The listing builds one solid part. Answer for the finished solid, in the listing's coordinates (mm). Face numbers are marked on the shaded views. A direction names the side the tool comes from. Coordinates: 2 decimals unless noted, no trailing zeros. Order: outer loops, then holes, each group sorted by start corner. A loop starts at its lowest first (then second) coordinate and runs counter-clockwise, first axis right, second up. Notation, with made-up numbers: M 63,38.25 L 93,38.25 A28 ccw 93,59.25 Z; hole C 80.5,37.25 d4. An arc over 180 degrees is marked long. One line per item, written item: value. Start each with the question number.
Q1. The part is cut by section D-D on x = 14.5. Give the vertices of the cut face in (y, z).
Q2. Determine the mould class of the marked faces 4 and 5 for opening direction X: pulls with the +X half, pulls with the -X half, needs draft (parallel to the pull), parting line crosses it, or undercut.
Q3. The part is cut by section A-A on y = 16. Give the vertices of the cut face in (x, z).
Q4. The part is cut by section C-C on y = -7. Give the vertices of the cut face in (x, z).
Q5. For the marked faces 1, 2 and 3, determine the directions among +Z, -Z, +X, -X, +Y, -Y from which every point of the face is accessible in a straight line to the end or side of a thin tool.
Q6. Straight lines are drawn through the part: line 1 along X through (y, z) = (-11.5, 4.5); line 2 along X through (y, z) = (-27.4, 16); line 3 along Y through (x, z) = (19.5, 6). For each, find the intervals that lie inside material, in ascending order. Write a range as [from, to].
Q7. Each of these flat-tipped pins is pushed along its axis until it touches: pin 1 Ø15.5 at (x, z) = (-20.5, 20) entering from +Y; pin 2 Ø10 at (y, z) = (-9.5, 12) entering from +X; pin 3 Ø2.5 at (x, z) = (16, 14.5) entering from -Y; pin 4 Ø8 at (x, z) = (0, 16) entering from -Y. Where does it stop, or does it pass through?
Q8. The part is cut by section B-B on z = 16. Give the number of separate pieces and of enclosed holes in the cut face, then the cut area to 3 significant figures.
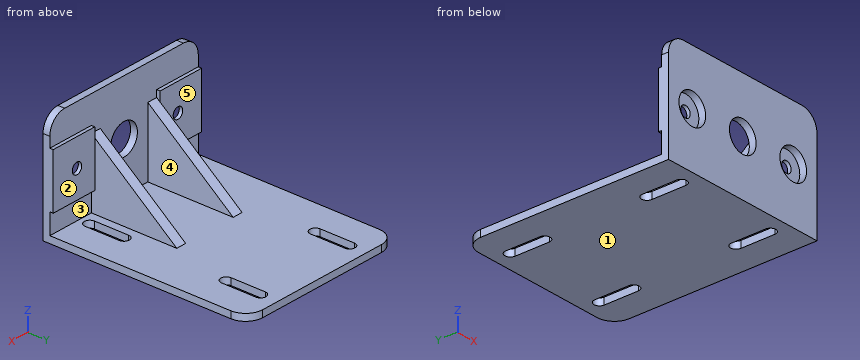
```python
from build123d import *

# Parameters (mm, degrees)
DODANIE_WYCI_GNI_CIE1_DEPTH = 2
WYTNIJ_WYCI_GNI_CIE1_REACH  = 41.102
SZKIC4_W                    = 50
SZKIC4_H                    = 2
DODANIE_WYCI_GNI_CIE2_DEPTH = 30
DODANIE_WYCI_GNI_CIE3_START = -14
DODANIE_WYCI_GNI_CIE3_DEPTH = 3
ZAOKR_GLENIE1_R             = 5
SZKIC7_R                    = 4.5
WYTNIJ_WYCI_GNI_CIE2_DEPTH  = 2
SZKIC8_W                    = 14
SZKIC8_H                    = 16
SZKIC8_R                    = 1.6
DODANIE_WYCI_GNI_CIE4_DEPTH = 1


with BuildPart() as part:
    # Szkic1 → Dodanie-wyci_gni_cie1 (new body)
    with BuildSketch(Plane.XY):
        with BuildLine():
            Line((-25, -30), (25, -30))
            Line((25, -30), (25, 25))
            ThreePointArc((25, 25), (23.535533906, 28.535533906), (20, 30))
            Line((20, 30), (-20, 30))
            ThreePointArc((-20, 30), (-23.535533906, 28.535533906), (-25, 25))
            Line((-25, 25), (-25, -30))
        make_face()
    extrude(amount=DODANIE_WYCI_GNI_CIE1_DEPTH)

    # Szkic2 → Wytnij-wyci_gni_cie1 (cut, up to next)
    with BuildSketch(Plane.XY.offset(2), mode=Mode.PRIVATE) as wytnij_wyci_gni_cie1_sk1:
        with BuildLine():
            Line((-13.4, 25), (-13.4, 15))
            ThreePointArc((-13.4, 15), (-15, 13.4), (-16.6, 15))
            Line((-16.6, 15), (-16.6, 25))
            ThreePointArc((-16.6, 25), (-15, 26.6), (-13.4, 25))
        make_face()
    wytnij_wyci_gni_cie1_tool1 = extrude(wytnij_wyci_gni_cie1_sk1.sketch, amount=-WYTNIJ_WYCI_GNI_CIE1_REACH, mode=Mode.PRIVATE) & part.part
    # Szkic2 → Wytnij-wyci_gni_cie1 (cut, up to next)
    with BuildSketch(Plane.XY.offset(2), mode=Mode.PRIVATE) as wytnij_wyci_gni_cie1_sk2:
        with BuildLine():
            Line((13.4, 25), (13.4, 15))
            ThreePointArc((13.4, 15), (15, 13.4), (16.6, 15))
            Line((16.6, 15), (16.6, 25))
            ThreePointArc((16.6, 25), (15, 26.6), (13.4, 25))
        make_face()
    wytnij_wyci_gni_cie1_tool2 = extrude(wytnij_wyci_gni_cie1_sk2.sketch, amount=-WYTNIJ_WYCI_GNI_CIE1_REACH, mode=Mode.PRIVATE) & part.part
    # Szkic2 → Wytnij-wyci_gni_cie1 (cut, up to next)
    with BuildSketch(Plane.XY.offset(2), mode=Mode.PRIVATE) as wytnij_wyci_gni_cie1_sk3:
        with BuildLine():
            Line((13.4, -25), (13.4, -15))
            ThreePointArc((13.4, -15), (15, -13.4), (16.6, -15))
            Line((16.6, -15), (16.6, -25))
            ThreePointArc((16.6, -25), (15, -26.6), (13.4, -25))
        make_face()
    wytnij_wyci_gni_cie1_tool3 = extrude(wytnij_wyci_gni_cie1_sk3.sketch, amount=-WYTNIJ_WYCI_GNI_CIE1_REACH, mode=Mode.PRIVATE) & part.part
    # Szkic2 → Wytnij-wyci_gni_cie1 (cut, up to next)
    with BuildSketch(Plane.XY.offset(2), mode=Mode.PRIVATE) as wytnij_wyci_gni_cie1_sk4:
        with BuildLine():
            Line((-13.4, -25), (-13.4, -15))
            ThreePointArc((-13.4, -15), (-15, -13.4), (-16.6, -15))
            Line((-16.6, -15), (-16.6, -25))
            ThreePointArc((-16.6, -25), (-15, -26.6), (-13.4, -25))
        make_face()
    wytnij_wyci_gni_cie1_tool4 = extrude(wytnij_wyci_gni_cie1_sk4.sketch, amount=-WYTNIJ_WYCI_GNI_CIE1_REACH, mode=Mode.PRIVATE) & part.part
    add(wytnij_wyci_gni_cie1_tool1.solids().sort_by_distance((-15, 20, 2))[0], mode=Mode.SUBTRACT)
    add(wytnij_wyci_gni_cie1_tool2.solids().sort_by_distance((15, 20, 2))[0], mode=Mode.SUBTRACT)
    add(wytnij_wyci_gni_cie1_tool3.solids().sort_by_distance((15, -20, 2))[0], mode=Mode.SUBTRACT)
    add(wytnij_wyci_gni_cie1_tool4.solids().sort_by_distance((-15, -20, 2))[0], mode=Mode.SUBTRACT)

    # Szkic4 → Dodanie-wyci_gni_cie2 (add)
    with BuildSketch(Plane.XY.offset(2)):
        with Locations((0, -29)):
            Rectangle(SZKIC4_W, SZKIC4_H)
    extrude(amount=DODANIE_WYCI_GNI_CIE2_DEPTH)


with BuildPart() as body_2:
    # Szkic6 → Dodanie-wyci_gni_cie3 (new body)
    with BuildSketch(Plane.ZY.offset(25).offset(DODANIE_WYCI_GNI_CIE3_START)):
        Polygon((2, -28), (2, -3), (22, -28), align=None)
    dodanie_wyci_gni_cie3 = extrude(amount=-DODANIE_WYCI_GNI_CIE3_DEPTH)


with BuildPart() as part_1:
    add(part.part)

    # Lustro3: Dodanie-wyci_gni_cie3 across plane
    add(dodanie_wyci_gni_cie3.mirror(Plane(origin=(0, 0, 0), x_dir=(0, 0, 1), z_dir=(1, 0, 0))))

    # Zaokr_glenie1
    zaokr_glenie1_edges = [part_1.edges().sort_by_distance(p)[0] for p in [
        (-25, -29, 32),
        (25, -29, 32),
    ]]
    fillet(zaokr_glenie1_edges, radius=ZAOKR_GLENIE1_R)

    # Szkic7 → Wytnij-wyci_gni_cie2 (cut)
    with BuildSketch(Plane.XZ.offset(30)):
        with Locations(Location((0, 16, 0), (0, 0, 270))):
            Circle(SZKIC7_R)
        with Locations(Location((-17, 16, 0), (0, 0, 270))):
            Circle(SZKIC7_R)
        with Locations(Location((17, 16, 0), (0, 0, 270))):
            Circle(SZKIC7_R)
    extrude(amount=-WYTNIJ_WYCI_GNI_CIE2_DEPTH, mode=Mode.SUBTRACT)

    add(body_2.part)  # Dodanie-wyci_gni_cie4 merges body 2
    # Szkic8 → Dodanie-wyci_gni_cie4 (add)
    # profile 1 of 2: a face of its own
    with BuildSketch(Plane(origin=(0, -28, 0), x_dir=(1, 0, 0), z_dir=(0, 1, 0))):
        with Locations((-18, -16)):
            Rectangle(SZKIC8_W, SZKIC8_H)
        with Locations(Location((-17, -16, 0), (0, 0, 270))):
            Circle(SZKIC8_R, mode=Mode.SUBTRACT)
    # profile 2 of 2: a face of its own
    with BuildSketch(Plane(origin=(0, -28, 0), x_dir=(1, 0, 0), z_dir=(0, 1, 0))):
        with Locations((18, -16)):
            Rectangle(SZKIC8_W, SZKIC8_H)
        with Locations(Location((17, -16, 0), (0, 0, 90))):
            Circle(SZKIC8_R, mode=Mode.SUBTRACT)
    extrude(amount=DODANIE_WYCI_GNI_CIE4_DEPTH)


solid = part_1.part
```
Output:
1. outline: M -30,0 L -26.52,0 L -26.52,2 L -28,2 L -28,8 L -27,8 L -27,24 L -28,24 L -28,32 L -30,32 L -30,19.74 L -28,19.74 L -28,12.26 L -30,12.26 Z; M -13.48,0 L 13.48,0 L 13.48,2 L -13.48,2 Z; M 26.52,0 L 30,0 L 30,2 L 26.52,2 Z
2. face 4: undercut
2. face 5: needs draft
3. outline: M -25,0 L -16.6,0 L -16.6,2 L -25,2 Z; M -13.4,0 L 13.4,0 L 13.4,2 L -13.4,2 Z; M 16.6,0 L 25,0 L 25,2 L 16.6,2 Z
4. outline: M -25,0 L 25,0 L 25,2 L 11,2 L 11,5.2 L 8,5.2 L 8,2 L -8,2 L -8,5.2 L -11,5.2 L -11,2 L -25,2 Z
5. face 1: -Z, +X, -X, +Y, -Y
5. face 2: +Z, +X, +Y
5. face 3: +X, +Y
6. line 1: x = [-11, -8], [8, 11]
6. line 2: x = [-25, -18.6], [-15.4, -8], [8, 15.4], [18.6, 25]
6. line 3: y = [-30, -28]
7. pin 1: stops at y = -27
7. pin 2: stops at x = 11
7. pin 3: stops at y = -28
7. pin 4: passes through
8. separate pieces: 4
8. enclosed holes: 0
8. area: 113 mm^2
